The listing builds one solid part. Answer for the finished solid, in the listing's coordinates (mm). Round coordinates to 2 decimals unless told otherwise and drop trailing zeros. Write each loop counter-clockwise with the first axis right and the second up, starting at its lowest first coordinate (ties: lowest second). Pieces come first, ordered by that corner, then holes. Notation, with made-up numbers: M 50,63 L 78,63 A16 ccw 78,76 Z; hole C 84,80.25 d9. An arc over 180 degrees is marked long. Write each question's results on one line, items separated by ' | '.
from build123d import *

# Parameters (mm, degrees)
F0_R     = 12.7
F1_DEPTH = 12.7


with BuildPart() as f1:
    # F0 (on Right) → F1 (new body, symmetric)
    with BuildSketch(Plane.YZ):
        with BuildLine():
            ThreePointArc((-45.452309, -44.795775), (24.206988, -59.047401), (63.816721, 0))
            ThreePointArc((63.816721, 0), (-22.773388, 59.614987), (-47.563074, -42.547948))
            ThreePointArc((-47.563074, -42.547948), (-41.266422, -22.971946), (-24.618088, -35.042599))
            ThreePointArc((-24.618088, -35.042599), (-31.933601, -46.544655), (-45.452309, -44.795775))
        make_face()
        with Locations((31.913808, -39.524028)):
            Circle(F0_R, mode=Mode.SUBTRACT)
        with Locations((-46.723463, 19.569239)):
            Circle(F0_R, mode=Mode.SUBTRACT)
        with Locations((0, 50.8)):
            Circle(F0_R, mode=Mode.SUBTRACT)
        with Locations((48.134091, 16.240359)):
            Circle(F0_R, mode=Mode.SUBTRACT)
    extrude(amount=F1_DEPTH, both=True)


solid = f1.part
1) Section D-D (z = 14.5) is taken. Determine the outline of the cut face in (x, y).
Return value:
outline: M -12.7,-62.15 L 12.7,-62.15 L 12.7,-58.37 L -12.7,-58.37 Z; M -12.7,-35.08 L 12.7,-35.08 L 12.7,35.55 L -12.7,35.55 Z; M -12.7,60.71 L 12.7,60.71 L 12.7,62.15 L -12.7,62.15 Z
2) Section C-C (x = 3.5) is taken. Determine the outline of the cut face in (y, z), then the cut area to 3 significant figures.
Return value:
outline: M -47.56,-42.55 A12.7 cw long -45.45,-44.8 A63.82 ccw long Z; hole C -46.72,19.57 d25.4; hole C 0,50.8 d25.4; hole C 31.91,-39.52 d25.4; hole C 48.13,16.24 d25.4 | area: 10,300 mm²
3) Each of these flat-tipped pins is pushed along its axis until it touches: pin 1 (3 mm diameter, centred on x = 6, y = -33.5, fed in from -Z); pin 2 (1.5 mm diameter, centred on x = 5.5, z = 48.5, fed in from -Y); pin 3 (3 mm diameter, centred on x = -1, z = 8, fed in from +Y). Where does it stop, or does it pass through?
Return value:
pin 1: z = -55.21 | pin 2: y = -42.34 | pin 3: y = 63.48
4) The mould has two halves that part along Y. Classify faces 1 (the face through (-12.7, -1, 1)), 2 (the face through (-0.18, -49.48, 7.17)): +Y half, -Y half, draft (parallel to the pull), parting line (faces both ways), or undercut.
Return value:
face 1: draft | face 2: undercut
5) Section B-B (z = 50.8) is taken. Determine the outline of the cut face in (x, y), then the cut area to 3 significant figures.
Return value:
outline: M -12.7,-38.63 L 12.7,-38.63 L 12.7,-12.7 L -12.7,-12.7 Z; M -12.7,12.7 L 12.7,12.7 L 12.7,38.63 L -12.7,38.63 Z | area: 1,320 mm²
6) Find the intervals of material crossed by line 1 (Z direction, x = -4.25, y = 0); line 2 (Y direction, x = 2.5, z = 20.5); line 3 (Y direction, x = -0.75, z = 26), in increasing order.
Return value:
line 1: -63.82 to 38.1, 63.5 to 63.82 | line 2: -60.43 to -59.39, -34.06 to 36.17, 60.1 to 60.43 | line 3: -58.28 to -57.67, -35.77 to 40.01, 56.26 to 58.28
7) Section A-A (y = 0) is taken. Determine the outline of the cut face in (x, z), then the cut area to 3 significant figures.
Return value:
outline: M -12.7,-63.82 L 12.7,-63.82 L 12.7,38.1 L -12.7,38.1 Z; M -12.7,63.5 L 12.7,63.5 L 12.7,63.82 L -12.7,63.82 Z | area: 2,600 mm²
